For this review, use the dimensioned drawing (mm, ordinates from the lowest corner) and the shaded views. A direction names the side the tool comes from. Round coordinates to 2 decimals unless told otherwise and drop trailing zeros. Write each loop counter-clockwise with the first axis right and the second up, starting at its lowest first coordinate (ties: lowest second). Pieces come first, ordered by that corner, then holes. Notation, with made-up numbers: M 31.25,-32 L 85.25,-32 A16 cw 85.25,-13 Z; hole C 3.5,-39 d5. An arc over 180 degrees is marked long. Use one line per item in the form item = value. Start each with the question number.
Item 1: For line 1 (Z direction, x = 4, y = 8); line 2 (Y direction, x = 6, z = 20); line 3 (Y direction, x = 6.25, z = 4.5), list the stretches that pass through material, from the lowest coordinate up. Write a range as [from, to].
Item 2: Add section D-D (z = 16.5). State the section outline as (x, y) points.
Item 3: Add section C-C (z = 20.5). State the section outline as (x, y) points.
Item 4: For the marked faces 1, 2 and 3, list the 3-axis set-ups (+Z, -Z, +X, -X, +Y, -Y) from which the entire face can be reached by the end or side of a thin tool; tool diameter is ignored.
Item 5: Add section A-A (x = 6). State the section outline as (y, z) points.
Item 6: For P1, Ø1.5, axis at y = 5, z = 14.5, coming from the +X side; P2, Ø5, axis at y = 1.5, z = 20, coming from the +X side; P3, Ø4, axis at x = 10.5, z = 11, coming from the -Y side; P4, Ø3.5, axis at x = 4, y = 6.5, coming from the -Z side, all flat-tipped, find the tip position at first contact; note any pin that passes through.
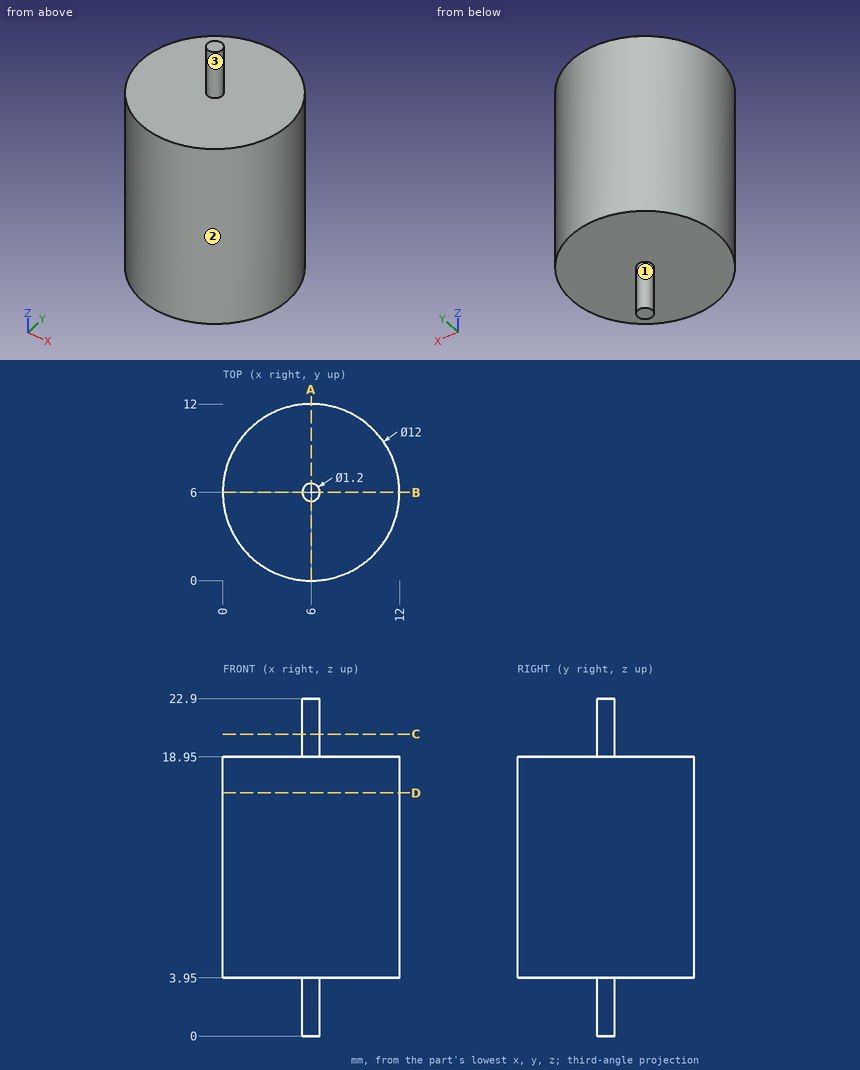
Calculated:
q1.line_1 = [3.95, 18.95]
q1.line_2 = [5.4, 6.6]
q1.line_3 = [0.01, 11.99]
q2.outline = C 6,6 d12
q3.outline = C 6,6 d1.2
q4.face_1 = -Z
q4.face_2 = +Z, -Z
q4.face_3 = +Z
q5.outline = M 0,3.95 L 5.4,3.95 L 5.4,0 L 6.6,0 L 6.6,3.95 L 12,3.95 L 12,18.95 L 6.6,18.95 L 6.6,22.9 L 5.4,22.9 L 5.4,18.95 L 0,18.95 Z
q6.P1 = 11.99
q6.P2 = 11.57
q6.P3 = 0.55
q6.P4 = 0
